Verification items for the finished model (mm, model axes). A direction names the side the tool comes from. Give positions to 0.01 mm unless a question says otherwise; leave off trailing zeros. Write each loop counter-clockwise with the first axis right and the second up, starting at its lowest first coordinate (ties: lowest second). Pieces come first, ordered by that corner, then holes. Notation, with made-up numbers: M 70,52.25 L 82,52.25 A19 cw 82,88.25 Z; hole C -28.5,37 d6. An arc over 180 degrees is marked long. Answer as a JSON object with one key per item and string values.
Autodesk Inventor part; units mm, degrees
ref_plane "YZ Plane" through (0, 0, 0) normal (1, 0, 0) x (0, 1, 0)
ref_plane "XZ Plane" through (0, 0, 0) normal (0, 1, 0) x (-1, 0, 0)
ref_plane "XY Plane" through (0, 0, 0) normal (0, 0, 1) x (1, 0, 0)
sketch "Sketch1" plane through (0, 0, 0) normal (0, 1, 0) x (-1, 0, 0)
  circle A0 centre (0, 0) radius 11
  circle A1 centre (0, 0) radius 5
  circle A2 centre (0, 0) radius 2
  line L0 (0, 0) -> (0, -8)
  line L1 (0, 0) -> (0, 8)
  circle A3 centre (0, 8) radius 1.5
  circle A4 centre (0, -8) radius 1.5
  circle A5 centre (-8, 0) radius 1.5
  circle A6 centre (0, -8) radius 1.5
  circle A7 centre (8, 0) radius 1.5
  dimension "d0" = 22
  dimension "d1" = 10
  dimension "d2" = 4
  dimension "d3" = 8
  dimension "d4" = 8
  dimension "d5" = 3
  dimension "d6" = 3
  dimension "d9" = 360
extrude "Extrusion1" add sketch "Sketch1" along normal blind 2
extrude "Extrusion2" add sketch "Sketch1" along normal blind 12 contours A1 L0 A2 L1 | L1 A2 L0 A1
sketch "Sketch2" plane through (0, 0, 0) normal (0, 0, 1) x (1, 0, 0)
  circle A0 centre (0, 7.0307) radius 1.5
  point P0 (0, 0)
  dimension "d15" = 3
extrude "Extrusion3" cut sketch "Sketch2" along normal mid plane 12
sketch "Sketch3" plane through (0, 0, 0) normal (0, -1, 0) x (1, 0, 0)
  circle A0 centre (0, 0) radius 2
  circle A1 centre (-8, 0) radius 1.5
  circle A2 centre (-8, 0) radius 1.5
  circle A3 centre (0, -8) radius 1.5
  circle A4 centre (0, -8) radius 1.5
  circle A5 centre (8, 0) radius 1.5
  circle A6 centre (8, 0) radius 1.5
  circle A7 centre (0, 8) radius 1.5
  circle A8 centre (0, 8) radius 1.5
  circle A9 centre (0, 0) radius 11.0573
properties part number "hub 4mm" material "Copper"
1) Thickness scan on L1, parallel to Z at x = 0, y = 1.5; L2, parallel to Y at x = 0, z = -3.25; L3, parallel to Y at x = 7.5, z = -5. Record the ranges inside material, lowest first.
Completed:
{"L1": "z = -11 to -9.5, -6.5 to -2, 2 to 6.5, 9.5 to 11", "L2": "y = 0 to 5.53, 8.53 to 12", "L3": "y = 0 to 2"}
2) Section check B-B on z = -0.5. Record the boundary of the cut face in (x, y).
Completed:
{"outline": "M -10.99,0 L -9.41,0 L -9.41,2 L -10.99,2 Z; M -6.59,0 L -1.94,0 L -1.94,12 L -4.97,12 L -4.97,2 L -6.59,2 Z; M 1.94,0 L 6.59,0 L 6.59,2 L 4.97,2 L 4.97,12 L 1.94,12 Z; M 9.41,0 L 10.99,0 L 10.99,2 L 9.41,2 Z"}
3) Release check for a two-part mould opening along Z. For faces 1 (the face through (-2.2, 12, 0.1)), 2 (the face through (2.38, 0.99, 10.74)), 3 (the face through (1.474, 5.916, -1.352)) record: pulls with the +Z half, pulls with the -Z half, needs draft (parallel to the pull), parting line crosses it, or undercut.
Completed:
{"face 1": "needs draft", "face 2": "parting line crosses it", "face 3": "undercut"}
4) Go/stop test with flat-tipped pins: pin 1 (2 mm diameter, centred on x = -1.5, y = 9.5, fed in from -Z); pin 2 (4 mm diameter, centred on x = -6, y = 6, fed in from -Z); pin 3 (6 mm diameter, centred on x = -1.5, y = 1.5, fed in from -Z); pin 4 (5 mm diameter, centred on x = -8, z = 0, fed in from +Y). Record where each tip stops, or that it passes through.
Completed:
{"pin 1": "stops at z = -4.97", "pin 2": "stops at z = -3", "pin 3": "stops at z = -11", "pin 4": "stops at y = 2"}
5) Access from +Z, -Z, +X, -X, +Y, -Y to the whole of each face (thin tool, end or side, straight path). Record for faces 4 (the face through (-2.307, 6.93, 4.436)), 5 (the face through (9.5, 0.99, -0.07)).
Completed:
{"face 4": "+Y", "face 5": "+Y, -Y"}
6) Section check C-C on x = 8. Record the boundary of the cut face in (y, z).
Completed:
{"outline": "M 0,-7.55 L 2,-7.55 L 2,-1.5 L 0,-1.5 Z; M 0,1.5 L 2,1.5 L 2,7.55 L 0,7.55 Z"}
7) Section check A-A on x = 0. Record the boundary of the cut face in (y, z), and give its area (3 significant figures).
Completed:
{"outline": "M 0,-11 L 2,-11 L 2,-9.5 L 0,-9.5 Z; M 0,-6.5 L 2,-6.5 L 2,-5 L 5.53,-5 L 5.53,-2 L 0,-2 Z; M 0,2 L 5.53,2 L 5.53,5 L 2,5 L 2,6.5 L 0,6.5 Z; M 0,9.5 L 2,9.5 L 2,11 L 0,11 Z; M 8.53,-5 L 12,-5 L 12,-2 L 8.53,-2 Z; M 8.53,2 L 12,2 L 12,5 L 8.53,5 Z", "area": "66.0 mm2"}
8) Section check D-D on z = -8. Record the boundary of the cut face in (x, y), and give its area (3 significant figures).
Completed:
{"outline": "M -7.55,0 L -1.5,0 L -1.5,2 L -7.55,2 Z; M 1.5,0 L 7.55,0 L 7.55,2 L 1.5,2 Z", "area": "24.2 mm2"}
